Here's how the part is built. I have some questions about the finished solid (model axes, mm). Round coordinates to 2 decimals unless told otherwise and drop trailing zeros. Order: outer loops, then holes, each group sorted by start corner. A loop starts at its lowest first (then second) coordinate and runs counter-clockwise, first axis right, second up. Notation, with made-up numbers: (70.25, -20) -> (104.25, -20) arc R27 cw to (104.25, -3) -> close; hole circle Ø10 at (79, 72.5). An arc over 180 degrees is marked (long way). Use a Markdown table: item, result. Add a question column.
from build123d import *

# Parameters (mm, degrees)
SKETCH_1_R      = 2
EXTRUDE_1_DEPTH = 2.5
FILLET_1_R      = 1


with BuildPart() as part:
    # 草图1 → 凸台-拉伸1 (new body)
    with BuildSketch(Plane(origin=(0, 0, 0), x_dir=(1, 0, 0), z_dir=(0, 1, 0))):
        with BuildLine():
            Line((29.554766525, 4.641792145), (29.554766525, 7.641792145))
            Line((29.554766525, 7.641792145), (29.554766525, 42.641792145))
            ThreePointArc((29.554766525, 42.641792145), (29.847659744, 43.348898926), (30.554766525, 43.641792145))
            Line((30.554766525, 43.641792145), (46.140552963, 43.641792145))
            ThreePointArc((46.140552963, 43.641792145), (46.523236395, 43.565671677), (46.847659744, 43.348898926))
            Line((46.847659744, 43.348898926), (51.261873307, 38.934685364))
            ThreePointArc((51.261873307, 38.934685364), (51.478646058, 38.610262015), (51.554766525, 38.227578582))
            Line((51.554766525, 38.227578582), (51.554766525, 31.641792145))
            Line((51.554766525, 31.641792145), (51.554766525, 15.641792145))
            Line((51.554766525, 15.641792145), (51.554766525, 9.056005707))
            ThreePointArc((51.554766525, 9.056005707), (51.478646058, 8.673322275), (51.261873307, 8.348898926))
            Line((51.261873307, 8.348898926), (46.847659744, 3.934685364))
            ThreePointArc((46.847659744, 3.934685364), (46.523236395, 3.717912612), (46.140552963, 3.641792145))
            Line((46.140552963, 3.641792145), (30.554766525, 3.641792145))
            ThreePointArc((30.554766525, 3.641792145), (29.847659744, 3.934685364), (29.554766525, 4.641792145))
        make_face()
        with Locations(Location((46.554766525, 10.641792145, 0), (0, 0, 270))):
            Circle(SKETCH_1_R, mode=Mode.SUBTRACT)
        with Locations(Location((46.554766525, 36.641792145, 0), (0, 0, 270))):
            Circle(SKETCH_1_R, mode=Mode.SUBTRACT)
    extrude(amount=EXTRUDE_1_DEPTH)

    # 圆角1
    fillet_1_edges = [part.edges().sort_by_distance(p)[0] for p in [
        (29.847659744, 2.5, -3.934685364),
        (29.847659744, 0, -43.348898926),
        (38.347659744, 0, -43.641792145),
        (46.523236395, 0, -43.565671677),
        (49.054766525, 0, -41.141792145),
        (51.478646058, 0, -38.610262015),
        (51.554766525, 0, -23.641792145),
        (38.347659744, 2.5, -3.641792145),
        (51.478646058, 0, -8.673322275),
        (49.054766525, 0, -6.141792145),
        (46.523236395, 0, -3.717912612),
        (38.347659744, 0, -3.641792145),
        (29.847659744, 0, -3.934685364),
        (29.554766525, 0, -23.641792145),
        (46.523236395, 2.5, -3.717912612),
        (49.054766525, 2.5, -6.141792145),
        (51.478646058, 2.5, -8.673322275),
        (51.554766525, 2.5, -23.641792145),
        (51.478646058, 2.5, -38.610262015),
        (49.054766525, 2.5, -41.141792145),
        (29.554766525, 2.5, -23.641792145),
        (46.523236395, 2.5, -43.565671677),
        (38.347659744, 2.5, -43.641792145),
        (29.847659744, 2.5, -43.348898926),
    ]]
    fillet(fillet_1_edges, radius=FILLET_1_R)


solid = part.part
(1) I'm going to push a flat-ended pin straight in: P1, Ø2, axis at x = 46.5, z = -11, coming from the -Y side. Where does the tip first touch, or does it pass through?
(2) I want a section at D-D on y = 0.6. List the corners of the cut face in (x, z) for me, and give its area (3 significant figures).
(3) Please list where these lines run through material, in increasing order: probe 1 along Z at (x, y) = (46, 0.75); probe 2 along Z at (x, y) = (46, 0.45); probe 3 along Y at (x, z) = (30.5, -34.5). Write a range as from..to.
(4) I want a section at C-C on z = -37.5. List the corners of the cut face in (x, y) for me, and give its area (3 significant figures).
(5) If we mould it in two halves opening along X, with no side actions, what happens to faces 1 (the cylindrical face through (44.78, 1.23, -9.72)), 2 (the cylindrical face through (29.8, 1.2, -43.3)), 3 (the cylindrical face through (44.78, 1.23, -35.72)), 4 (the flat face through (49.024, 1.246, -41.173))? For each: pulls with the +X half, pulls with the -X half, needs draft (parallel to the pull), parting line crosses it, or undercut.
(6) I want a section at A-A on z = -29. List the corners of the cut face in (x, y) for me.
(7) I want a section at B-B on x = 45.5. List the corners of the cut face in (y, z) for me, and give its area (3 significant figures).
Output:
| question | item | result |
|---|---|---|
| 1 | P1 | through |
| 2 | outline | (29.64, -42.64) arc R0.92 ccw to (30.55, -43.56) -> (46.14, -43.56) arc R0.92 ccw to (46.79, -43.29) -> (51.2, -38.88) arc R0.92 ccw to (51.47, -38.23) -> (51.47, -9.06) arc R0.92 ccw to (51.2, -8.41) -> (46.79, -3.99) arc R0.92 ccw to (46.14, -3.73) -> (30.55, -3.73) arc R0.92 ccw to (29.64, -4.64) -> close; hole circle Ø4 at (46.55, -36.64); hole circle Ø4 at (46.55, -10.64) |
| 2 | area | 820 mm² |
| 3 | probe 1 | -43.61..-38.56, -34.72..-12.56, -8.72..-3.67 |
| 3 | probe 2 | -43.48..-38.56, -34.72..-12.56, -8.72..-3.81 |
| 3 | probe 3 | 0..2.5 |
| 4 | outline | (29.55, 1) arc R1 ccw to (30.55, 0) -> (44.75, 0) -> (44.75, 2.5) -> (30.55, 2.5) arc R1 ccw to (29.55, 1.5) -> close; (48.36, 0) -> (50.55, 0) arc R1 ccw to (51.55, 1) -> (51.55, 1.5) arc R1 ccw to (50.55, 2.5) -> (48.36, 2.5) -> close |
| 4 | area | 45.1 mm² |
| 5 | face 1 | undercut |
| 5 | face 2 | pulls with the -X half |
| 5 | face 3 | undercut |
| 5 | face 4 | pulls with the +X half |
| 6 | outline | (29.55, 1) arc R1 ccw to (30.55, 0) -> (50.55, 0) arc R1 ccw to (51.55, 1) -> (51.55, 1.5) arc R1 ccw to (50.55, 2.5) -> (30.55, 2.5) arc R1 ccw to (29.55, 1.5) -> close |
| 7 | outline | (0, -42.64) arc R1 ccw to (1, -43.64) -> (1.5, -43.64) arc R1 ccw to (2.5, -42.64) -> (2.5, -38.34) -> (0, -38.34) -> close; (0, -34.94) -> (2.5, -34.94) -> (2.5, -12.34) -> (0, -12.34) -> close; (0, -8.94) -> (2.5, -8.94) -> (2.5, -4.64) arc R1 ccw to (1.5, -3.64) -> (1, -3.64) arc R1 ccw to (0, -4.64) -> close |
| 7 | area | 82.1 mm² |
